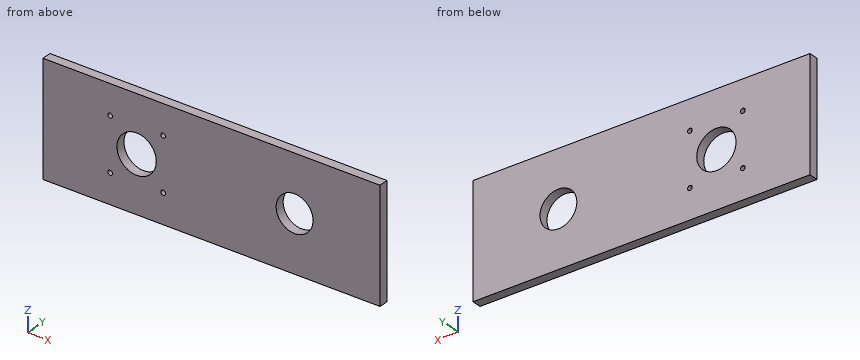
from build123d import *

# Parameters (mm, degrees)
SKETCH1_W             = 180
SKETCH1_H             = 60
SKETCH1_R             = 10.5
SKETCH1_R_2           = 9.848320848
BOSS_EXTRUDE1_DEPTH   = 5
M3X0_5_TAPPED_HOLE1_D = 2.5


with BuildPart() as part:
    # Sketch1 → Boss-Extrude1 (new body)
    with BuildSketch(Plane(origin=(0, 0, 0), x_dir=(1, 0, 0), z_dir=(0, 1, 0))):
        with Locations((40, 0)):
            Rectangle(SKETCH1_W, SKETCH1_H)
        with Locations(Location((0, 0, 0), (0, 0, 270))):
            Circle(SKETCH1_R, mode=Mode.SUBTRACT)
        with Locations(Location((84.38561279, 0, 0), (0, 0, 270))):
            Circle(SKETCH1_R_2, mode=Mode.SUBTRACT)
    extrude(amount=BOSS_EXTRUDE1_DEPTH)

    # M3x0.5 Tapped Hole1 (through all)
    with Locations(Plane(origin=(0, 5, 0), x_dir=(1, 0, 0), z_dir=(0, 1, 0))):
        with Locations((-14.142135624, 14.142135624), (14.142135624, 14.142135624), (14.142135624, -14.142135624), (-14.142135624, -14.142135624), (0, 0)):
            Hole(M3X0_5_TAPPED_HOLE1_D / 2)


solid = part.part
Design review of the part built by this model. Coordinates are the model's own, in mm. Coordinates: 2 decimals unless noted, no trailing zeros. Loops run counter-clockwise (first coordinate to the right, second up) from the corner with the lowest first, then second, coordinate; pieces in that order, holes last. Notation, with made-up numbers: M -10.5,-8 L -3.5,-8 A6 cw -3.5,-1 Z; hole C 38,24.25 d7. An arc over 180 degrees is marked long. Use one line per item in the form item = value.
(1) Consider section C-C (y = 2.95). Write out the cut boundary in (x, z).
Return value:
outline = M -50,-30 L 130,-30 L 130,30 L -50,30 Z; hole C -14.14,-14.14 d2.5; hole C -14.14,14.14 d2.5; hole C 0,0 d21; hole C 14.14,-14.14 d2.5; hole C 14.14,14.14 d2.5; hole C 84.39,0 d19.7
(2) Consider section B-B (x = 0). Write out the cut boundary in (y, z).
Return value:
outline = M 0,-30 L 5,-30 L 5,-10.5 L 0,-10.5 Z; M 0,10.5 L 5,10.5 L 5,30 L 0,30 Z
(3) Consider section A-A (z = 0). Write out the cut boundary in (x, y).
Return value:
outline = M -50,0 L -10.5,0 L -10.5,5 L -50,5 Z; M 10.5,0 L 74.54,0 L 74.54,5 L 10.5,5 Z; M 94.23,0 L 130,0 L 130,5 L 94.23,5 Z
(4) For line 1 along X through (y, z) = (2.85, 0); line 2 along X through (y, z) = (2.2, 6.5); line 3 along Z through (x, y) = (86, 3.1), list the stretches that pass through material, from the lowest coordinate up. Write a range as from..to.
Return value:
line_1 = -50..-10.5, 10.5..74.54, 94.23..130
line_2 = -50..-8.25, 8.25..76.99, 91.78..130
line_3 = -30..-9.72, 9.72..30
(5) Clearance check with a flat-ended pin moving along its axis: P1, Ø3, axis at x = -14.14, z = -14.14, coming from the +Y side. State where the tip first meets the part, or that it passes through.
Return value:
P1 = 5
